Geometry check sheet. Reference: drawing and pictorial views, mm from the part's lowest x, y, z. Round coordinates to 2 decimals unless told otherwise and drop trailing zeros. Order: outer loops, then holes, each group sorted by start corner. A loop starts at its lowest first (then second) coordinate and runs counter-clockwise, first axis right, second up.
(1) Cross-section at B-B on x = 27. Enter the section's corners in (y, z), and give its area (3 significant figures).
(2) Cross-section at C-C on x = 38. Enter the section's corners in (y, z).
(3) Thickness scan on L1, parallel to Z at x = 45.5, y = 34; L2, parallel to X at y = 26.5, z = 108.5; L3, parallel to Z at x = 31, y = 35. Record the ranges inside material, lowest first.
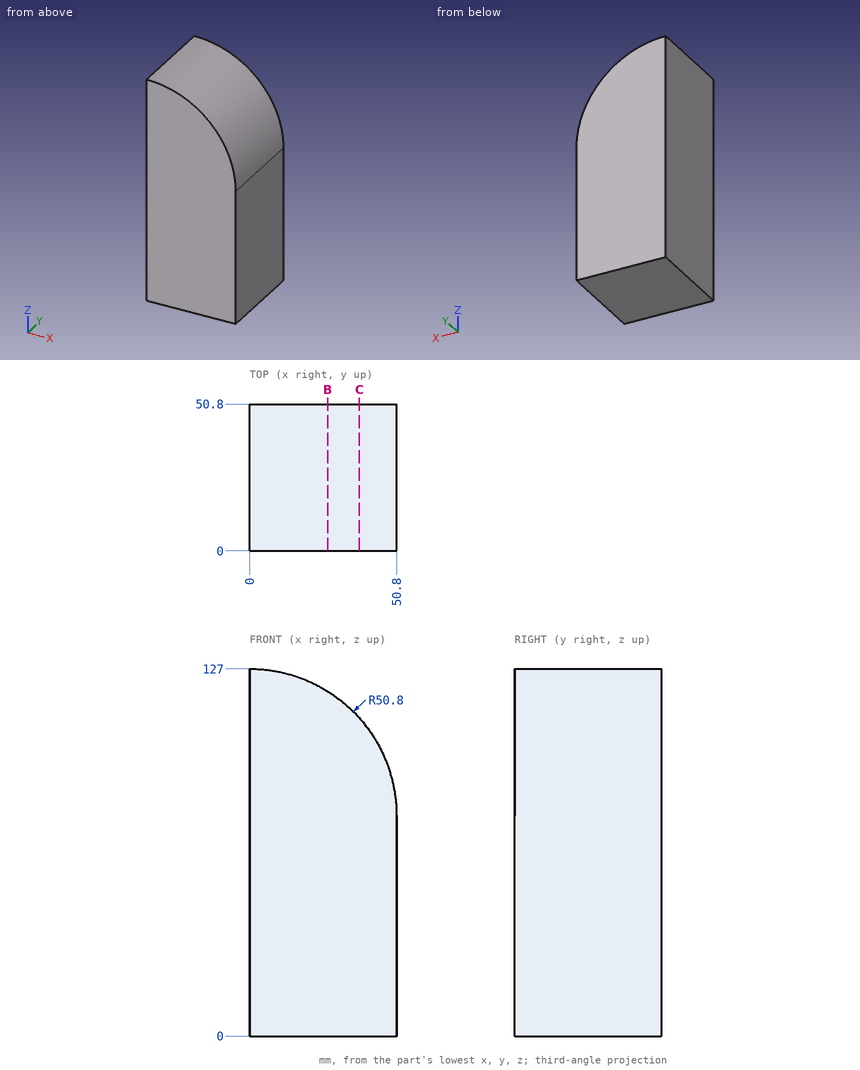
Found:
1. outline: (0, 0) - (50.8, 0) - (50.8, 119.23) - (0, 119.23) - close
1. area: 6,060 mm2
2. outline: (0, 0) - (50.8, 0) - (50.8, 109.91) - (0, 109.91) - close
3. L1: z = 0 to 98.79
3. L2: x = 0 to 39.21
3. L3: z = 0 to 116.44
